```python
from build123d import *

# Parameters (mm, degrees)
F0_R     = 17
F1_DEPTH = 5
F0_R_2   = 19
F0_W     = 22.5
F0_H     = 2
F2_DEPTH = 2
F3_DEPTH = 2
F4_DEPTH = 15


with BuildPart() as f1:
    # F0 (on Front) → F1 (new body)
    with BuildSketch(Plane.XZ):
        Circle(F0_R)
        Polygon((11.25, -9.25), (11.25, -11.25), (-11.25, -11.25), (-11.25, -9.25), (-11.25, 9.25), (-11.25, 11.25), (11.25, 11.25), (11.25, 9.25), align=None, mode=Mode.SUBTRACT)
    extrude(amount=F1_DEPTH)

    # F0 (on Front) → F2 (join)
    with BuildSketch(Plane.XZ):
        Circle(F0_R_2)
        Circle(F0_R, mode=Mode.SUBTRACT)
        Circle(F0_R)
        Polygon((11.25, -9.25), (11.25, -11.25), (-11.25, -11.25), (-11.25, -9.25), (-11.25, 9.25), (-11.25, 11.25), (11.25, 11.25), (11.25, 9.25), align=None, mode=Mode.SUBTRACT)
        with Locations((0, 10.25)):
            Rectangle(F0_W, F0_H)
        with Locations((0, -10.25)):
            Rectangle(F0_W, F0_H)
    extrude(amount=F2_DEPTH)

    # F0 (on Front) → F3 (join)
    with BuildSketch(Plane.XZ):
        with Locations((0, -10.25)):
            Rectangle(F0_W, F0_H)
    extrude(amount=F3_DEPTH)

    # F0 (on Front) → F4 (join)
    with BuildSketch(Plane.XZ):
        Circle(F0_R_2)
        Circle(F0_R, mode=Mode.SUBTRACT)
    extrude(amount=F4_DEPTH)


solid = f1.part
```
For this review, take the finished solid that the model builds, in its own axes (mm). A direction names the side the tool comes from. Give positions to 0.01 mm unless a question says otherwise; leave off trailing zeros. Order: outer loops, then holes, each group sorted by start corner. A loop starts at its lowest first (then second) coordinate and runs counter-clockwise, first axis right, second up.
1) Take a section at A-A (z = 0). Give the boundary of the cut face in (x, y), then the cut area to 4 significant figures.
2) Insertion check: pin 1 (1 mm diameter, centred on x = 4, z = -10.5, fed in from -Y); pin 2 (3 mm diameter, centred on x = 7.5, y = -11.5, fed in from +Z); pin 3 (0.9 mm diameter, centred on x = 3.5, y = -3.5, fed in from -Z). Each pin has a flat end and moves straight along its axis. Give the tip position at first contact, or say it passes through.
3) For faces 5 (the face through (0, -1, -9.25)), 6 (the face through (12, 0, 0)), 7 (the face through (0, -2, -10)), list the 3-axis set-ups (+Z, -Z, +X, -X, +Y, -Y) from which the entire face can be reached by the end or side of a thin tool; tool diameter is ignored.
4) Wall thickness on line 1 (Z direction, x = 0, y = -12); line 2 (Y direction, x = 14.5, z = -7.5); line 3 (X direction, y = -5.25, z = 7): over which ranges is each line inside the solid? List them lowest first.
5) Take a section at D-D (x = 7.5). Give the boundary of the cut face in (y, z).
6) The part is to be moulded in two halves that separate along X. For faces 1 (the face through (8.767, -7.395, -16.856)), 2 (the face through (0, -1, 9.25)), 3 (the face through (9.139, -9.93, 14.334)), 4 (the face through (-14, -15, -10)), say which applies: released by +X, released by -X, zero draft, split by the parting line, or undercut.
7) Take a section at C-C (y = -3.75). Give the boundary of the cut face in (x, z).
8) Take a section at B-B (x = 0). Give the boundary of the cut face in (y, z).
Derived:
1. outline: (-19, -15) - (-17, -15) - (-17, -5) - (-11.25, -5) - (-11.25, 0) - (-19, 0) - close; (11.25, -5) - (17, -5) - (17, -15) - (19, -15) - (19, 0) - (11.25, 0) - close
1. area: 117.5 mm2
2. pin 1: stops at y = -2
2. pin 2: stops at z = 18.03
2. pin 3: stops at z = -18.75
3. face 5: +Y, -Y
3. face 6: +Z, -Z, +X, -X, +Y
3. face 7: -Y
4. line 1: z = -19 to -17, 17 to 19
4. line 2: y = -5 to 0
4. line 3: x = -17.66 to -15.49, 15.49 to 17.66
5. outline: (-15, -17.46) - (0, -17.46) - (0, -9.25) - (-2, -9.25) - (-2, -11.25) - (-5, -11.25) - (-5, -15.26) - (-15, -15.26) - close; (-15, 15.26) - (-5, 15.26) - (-5, 11.25) - (-2, 11.25) - (-2, 9.25) - (0, 9.25) - (0, 17.46) - (-15, 17.46) - close
6. face 1: split by the parting line
6. face 2: undercut
6. face 3: undercut
6. face 4: zero draft
7. outline: circle Ø38 at (0, 0); hole (-11.25, -11.25) - (11.25, -11.25) - (11.25, 11.25) - (-11.25, 11.25) - close
8. outline: (-15, -19) - (0, -19) - (0, -9.25) - (-2, -9.25) - (-2, -11.25) - (-5, -11.25) - (-5, -17) - (-15, -17) - close; (-15, 17) - (-5, 17) - (-5, 11.25) - (-2, 11.25) - (-2, 9.25) - (0, 9.25) - (0, 19) - (-15, 19) - close
